Job drawing, mm, ordinate dimensions from the low corner. One solid piece. Give positions to 0.01 mm unless a question says otherwise; leave off trailing zeros. Loops run counter-clockwise (first coordinate to the right, second up) from the corner with the lowest first, then second, coordinate; pieces in that order, holes last. Notation, with made-up numbers: M 42,0.25 L 80,0.25 A19 ccw 80,4.25 Z; hole C -31.75,71.25 d11. An arc over 180 degrees is marked long. One line per question, with ' | ' between items.
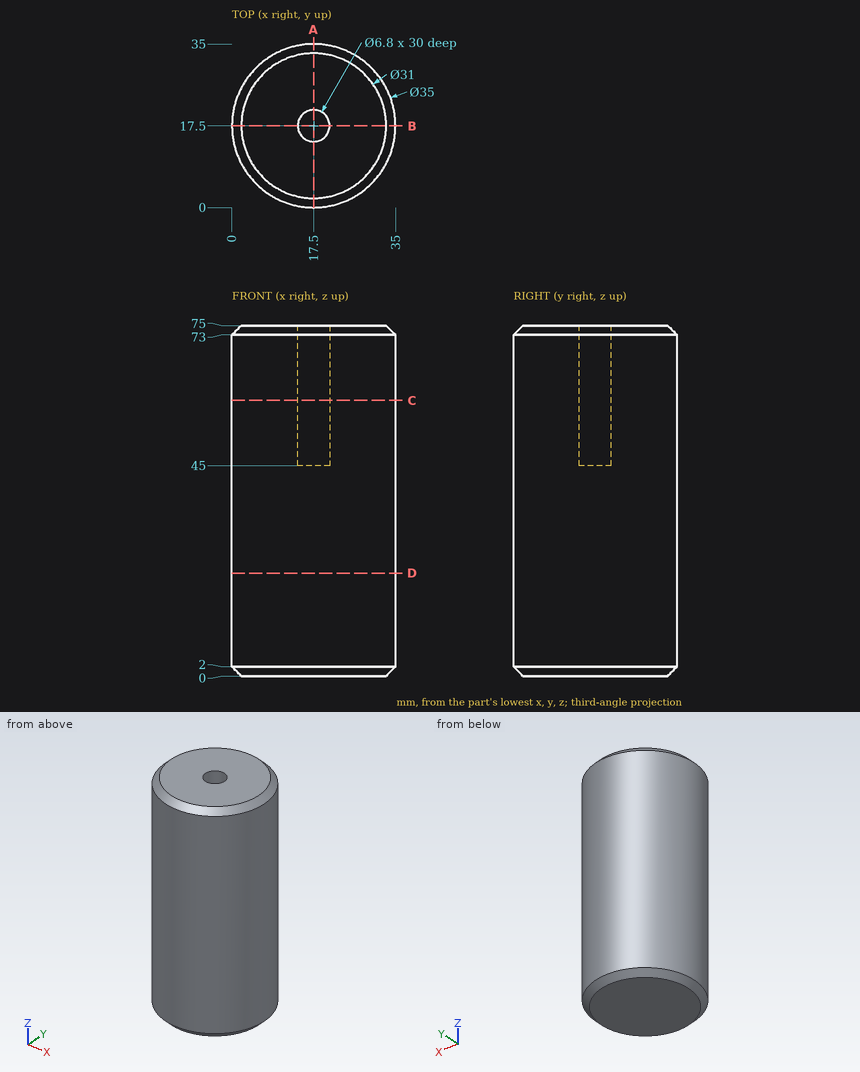
Item 1: Drill centre lines: line 1 along Y through (x, z) = (17.5, 54.75); line 2 along X through (y, z) = (15.5, 69); line 3 along X through (y, z) = (17, 46). Where is each one in solid material? Low to high. Write a range as [from, to].
Conclusion:
line 1: [0, 14.1], [20.9, 35] | line 2: [0.11, 14.75], [20.25, 34.89] | line 3: [0.01, 14.14], [20.86, 34.99]
Item 2: Drop flat-ended pins along their axis: P1, Ø1, axis at x = 10, z = 22.5, coming from the +Y side; P2, Ø2, axis at x = 31.5, y = 16.5, coming from the -Z side; P3, Ø4, axis at x = 20, z = 40, coming from the -Y side; P4, Ø2, axis at x = 20, z = 41.5, coming from the -Y side. Give the stop position or say it passes through.
Conclusion:
P1: y = 33.54 | P2: z = 0 | P3: y = 0.01 | P4: y = 0.06
Item 3: Saw through at C-C on z = 59. Give the cut face in (x, y).
Conclusion:
outline: C 17.5,17.5 d35; hole C 17.5,17.5 d6.8
Item 4: Saw through at D-D on z = 22. Give the cut face in (x, y).
Conclusion:
outline: C 17.5,17.5 d35
Item 5: Saw through at A-A on x = 17.5. Give the cut face in (y, z).
Conclusion:
outline: M 0,2 L 2,0 L 33,0 L 35,2 L 35,73 L 33,75 L 20.9,75 L 20.9,45 L 14.1,45 L 14.1,75 L 2,75 L 0,73 Z
